Autodesk Inventor part; units mm, degrees
ref_plane "YZ Plane" through (0, 0, 0) normal (1, 0, 0) x (0, 1, 0)
ref_plane "XZ Plane" through (0, 0, 0) normal (0, 1, 0) x (-1, 0, 0)
ref_plane "XY Plane" through (0, 0, 0) normal (0, 0, 1) x (1, 0, 0)
sketch "Sketch1" plane through (0, 0, 0) normal (0, 1, 0) x (-1, 0, 0)
  line L0 (-5.9, 0) -> (-1.25, 0)
  line L1 (-5.9, 0) -> (-5.9, 0.8)
  line L2 (-5.9, 0.8) -> (-1.25, 0.8)
  line L3 (0, 1.25) -> (0, 10.35)
  line L4 (0, 10.35) -> (-0.8, 10.35)
  line L5 (-0.8, 10.35) -> (-0.8, 1.25)
  arc A0 (-1.25, 0) -> (0, 1.25) centre (-1.25, 1.25) ccw
  arc A1 (-1.25, 0.8) -> (-0.8, 1.25) centre (-1.25, 1.25) ccw
  point P0 (0, 0)
  dimension "d0" = 0.8
  dimension "d1" = 10.35
  dimension "d2" = 5.9
  dimension "d3" = 1.25
extrude "Extrusion1" add sketch "Sketch1" along normal mid plane 6
sketch "Sketch2" plane through (0.8, -3, 1.25) normal (1, 0, 0) x (0, 0, -1)
  line L0 (-9.1, 0) -> (-9.1, 6)
  arc A0 (-4.3396, 1.918) -> (-4.3396, 4.082) centre (-3.95, 3) ccw
  arc A1 (-5.6783, 3.6) -> (-5.6783, 2.4) centre (-5.4623, 3) ccw
  line L1 (-5.6783, 3.6) -> (-4.3396, 4.082)
  line L2 (-5.6783, 2.4) -> (-4.3396, 1.918)
  line L3 (1.25, 6) -> (1.25, 0)
  line L4 (-9.1, 6) -> (-2.1, 6)
  line L5 (-2.1, 6) -> (-2.1, 5.375)
  line L6 (-2.1, 5.375) -> (-9.1, 5.375)
  line L7 (-9.1, 5.375) -> (-9.1, 6)
  line L8 (-9.1, 0) -> (-2.1, 0)
  line L9 (-2.1, 0) -> (-2.1, 0.625)
  line L10 (-2.1, 0.625) -> (-9.1, 0.625)
  line L11 (-9.1, 0.625) -> (-9.1, 0)
  point P0 (1.25, 3)
  point P1 (1.25, 3)
  dimension "d6" = 3
  dimension "d7" = 3.3
  dimension "d8" = 1.15
  dimension "d9" = 1.2
  dimension "d27" = 4.75
  dimension "d28" = 7
extrude "Extrusion2" cut sketch "Sketch2" against normal through all
chamfer "Chamfer1" distance 1.35 angle 45 2 edges at (5.9, 3, 0.4) (5.9, -3, 0.4)
chamfer "Chamfer2" distance 1.3 distance2 1.1 1 edges at (0.4, -2.375, 10.35) measured on face at (0.2667, -0.7917, 10.35)
chamfer "Chamfer3" distance 1.3 distance2 1.1 1 edges at (0.4, 2.375, 10.35) measured on face at (0.2667, 0.075, 10.35)
chamfer "Chamfer4" distance 0.3 distance2 0.95 1 edges at (0.8, 0, 10.35) measured on face at (0.2667, -0.3583, 10.35)
chamfer "Chamfer5" distance 0.3 distance2 0.95 1 edges at (0, 0, 10.35) measured on face at (0.1667, -0.3583, 10.35)
properties material "Nickel-Copper Alloy 400"
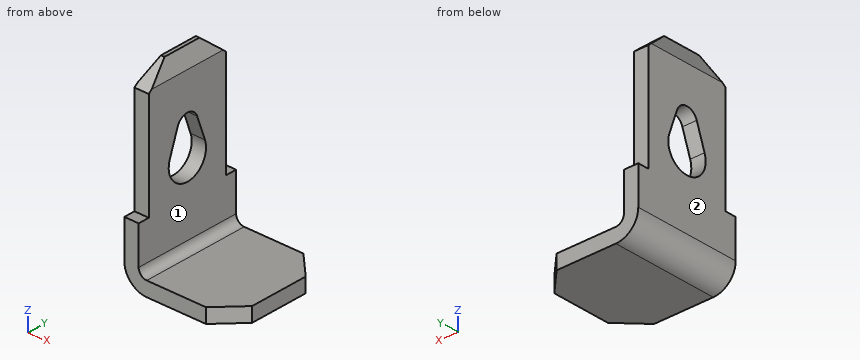
The listing builds one solid part. Answer for the finished solid, in the listing's coordinates (mm). Face numbers are marked on the shaded views. A direction names the side the tool comes from. Give positions to 0.01 mm unless a question says otherwise; leave off trailing zeros. Write each loop counter-clockwise with the first axis right and the second up, starting at its lowest first coordinate (ties: lowest second). Pieces come first, ordered by that corner, then holes. Notation, with made-up numbers: (75, 42) -> (105, 42) arc R25 cw to (105, 70) -> close; hole circle Ø11 at (-34, 78). An arc over 180 degrees is marked (long way). Write item = value, one per line. Start each with the question number.
1) The part is cut by section A-A, the plane z = 5.2. Determine the outline of the cut face in (x, y) (3 decimals), and give its area (3 significant figures).
2) Which of the six approach directions +Z, -Z, +X, -X, +Y, -Y give full straight-line access (tool end or side, diameter ignored) to the marked faces 1 and 2?
3) Straight lines are drawn through the part: line 1 along Y through (x, z) = (0.65, 5.2) (3 decimals); line 2 along X through (y, z) = (-0.05, 9.25). For each, find the intervals that lie inside material, in ascending order.
4) The part is cut by section B-B, the plane y = 2.5. Determine the outline of the cut face in (x, z), and give its area (3 significant figures).
5) The part is cut by section C-C, the plane y = 0. Determine the outline of the cut face in (x, z), and give its area (3 significant figures).
6) Each of these flat-tipped pins is pushed along its axis until it touches: pin 1 (3 mm diameter, centred on y = 0.5, z = 4, fed in from -X); pin 2 (0.9 mm diameter, centred on x = 0.5, z = 6, fed in from -Y) (3 decimals); pin 3 (1 mm diameter, centred on y = 1.5, z = 8, fed in from +X); pin 4 (0.5 mm diameter, centred on x = 0.5, y = -3, fed in from +Z). Where does it stop, or does it pass through?
7) The part is cut by section D-D, the plane x = 5.45. Determine the outline of the cut face in (y, z).
Solutions:
q1.outline = (0, -2.375) -> (0.8, -2.375) -> (0.8, -1.15) -> (0, -1.15) -> close; (0, 1.15) -> (0.8, 1.15) -> (0.8, 2.375) -> (0, 2.375) -> close
q1.area = 1.96 mm²
q2.face_1 = +Z, +X, +Y, -Y
q2.face_2 = +Z, -Z, -X, +Y, -Y
q3.line_1 = -2.375 to -1.15, 1.15 to 2.375
q3.line_2 = 0 to 0.8
q4.outline = (0, 1.25) arc R1.25 ccw to (1.25, 0) -> (5.05, 0) -> (5.05, 0.8) -> (1.25, 0.8) arc R0.45 cw to (0.8, 1.25) -> (0.8, 3.35) -> (0, 3.35) -> close
q4.area = 5.79 mm²
q5.outline = (0, 1.25) arc R1.25 ccw to (1.25, 0) -> (5.9, 0) -> (5.9, 0.8) -> (1.25, 0.8) arc R0.45 cw to (0.8, 1.25) -> (0.8, 4.05) -> (0, 4.05) -> close; (0, 7.35) -> (0.8, 7.35) -> (0.8, 9.4) -> (0.5, 10.35) -> (0.3, 10.35) -> (0, 9.4) -> close
q5.area = 9.14 mm²
q6.pin_1 = 0
q6.pin_2 = -2.375
q6.pin_3 = 0.8
q6.pin_4 = 3.35
q7.outline = (-2.1, 0) -> (2.1, 0) -> (2.1, 0.8) -> (-2.1, 0.8) -> close
